```python
from build123d import *

# Parameters (mm, degrees)
SKETCH_1_W          = 5
SKETCH_1_H          = 4
EXTRUDE_1_DEPTH     = 1.5
CHAMFER_1_SIZE      = 0.5
EXTRUDE_2_DEPTH     = 5
SKETCH_3_W          = 0.34
SKETCH_3_H          = 1.1
SKETCH_3_W_2        = 0.76
CUT_EXTRUDE_1_DEPTH = 5.35


with BuildPart() as part:
    # Эскиз1 → Бобышка-Вытянуть1 (new body)
    with BuildSketch(Plane(origin=(0, 0, 0), x_dir=(1, 0, 0), z_dir=(0, 1, 0))):
        Rectangle(SKETCH_1_W, SKETCH_1_H)
    extrude(amount=EXTRUDE_1_DEPTH)

    # Фаска1
    chamfer_1_edges = [part.edges().sort_by_distance(p)[0] for p in [
        (0, 1.5, 2),
    ]]
    chamfer(chamfer_1_edges, length=CHAMFER_1_SIZE)

    # Эскиз2 → Бобышка-Вытянуть2 (add, through all)
    with BuildSketch(Plane(origin=(2.5, 0, 0), x_dir=(0, 0, -1), z_dir=(1, 0, 0))):
        Polygon((-2, 0.75), (-2.25, 0.75), (-2.25, -0.1), (-3.1, -0.1), (-3.1, -0.25), (-2.1, -0.25), (-2.1, 0.6), (0, 0.6), (0, 0.75), align=None)
    extrude_2 = extrude(amount=-EXTRUDE_2_DEPTH)

    # Эскиз3 → Вырез-Вытянуть1 (cut, through all)
    with BuildSketch(Plane(origin=(0, 1.5, 0), x_dir=(1, 0, 0), z_dir=(0, 1, 0))):
        with Locations((-2.33, -2.55)):
            Rectangle(SKETCH_3_W, SKETCH_3_H)
        with Locations((-1.27, -2.55)):
            Rectangle(SKETCH_3_W_2, SKETCH_3_H)
        with Locations((0, -2.55)):
            Rectangle(SKETCH_3_W_2, SKETCH_3_H)
        with Locations((1.27, -2.55)):
            Rectangle(SKETCH_3_W_2, SKETCH_3_H)
        with Locations((2.33, -2.55)):
            Rectangle(SKETCH_3_W, SKETCH_3_H)
    cut_extrude_1 = extrude(amount=-CUT_EXTRUDE_1_DEPTH, mode=Mode.SUBTRACT)

    # Зеркальное отражение1: Бобышка-Вытянуть2, Вырез-Вытянуть1 across plane
    add(extrude_2.mirror(Plane.XY))
    add(cut_extrude_1.mirror(Plane.XY), mode=Mode.SUBTRACT)


solid = part.part
```
For this review, take the finished solid that the model builds, in its own axes (mm). A direction names the side the tool comes from. Round coordinates to 2 decimals unless told otherwise and drop trailing zeros. Write each loop counter-clockwise with the first axis right and the second up, starting at its lowest first coordinate (ties: lowest second). Pieces come first, ordered by that corner, then holes. Notation, with made-up numbers: (79.5, 82) - (127.5, 82) arc R18 ccw to (127.5, 86) - close; hole circle Ø9 at (21, 74). An arc over 180 degrees is marked (long way). Answer as CSV lines item,"result". Start each with the question number.
(1) Add section D-D, the plane y = 1.2. State the section outline as (x, z) points, plus the area to 3 significant figures.
(2) For line 1 (Z direction, x = 2.2, y = 0.6); line 2 (Y direction, x = -0.2, z = 0.5); line 3 (Z direction, x = -1.4, y = 1.45), list the stretches that pass through material, from the lowest coordinate up.
(3) Add section A-A, the plane x = -0.55. State the section outline as (y, z) points, plus the area to 3 significant figures.
(4) For pin 1 (0.8 mm diameter, centred on y = 0, z = -3, fed in from +X); pin 2 (0.5 mm diameter, centred on y = 0, z = -2.5, fed in from -X); pin 3 (0.8 mm diameter, centred on x = -0.5, y = 0.5, fed in from -Z), all flat-tipped, find the tip position at first contact; note any pin that passes through.
(5) Add section C-C, the plane z = -1.5. State the section outline as (x, y) points.
(6) Machinability: for faces 1 (the flat face through (0, 0, 0)), 2 (the flat face through (0, 1.5, 0)), which of the approach directions +Z, -Z, +X, -X, +Y, -Y give a long, thin tool a straight path to every point of the face, cutting with its end or side? Answer none if there is none.
(7) Add section B-B, the plane y = 0.15. State how many separate pieces and enclosed holes the cut face has, plus the area to 3 significant figures.
From the geometry:
1,outline,"(-2.5, -2) - (2.5, -2) - (2.5, 1.8) - (-2.5, 1.8) - close"
1,area,"19.0 mm²"
2,line 1,"z = -2 to 2"
2,line 2,"y = 0 to 1.5"
2,line 3,"z = -2 to 1.55"
3,outline,"(-0.25, -3.1) - (-0.1, -3.1) - (-0.1, -2.25) - (0.75, -2.25) - (0.75, -2) - (1.5, -2) - (1.5, 1.5) - (1, 2) - (0.75, 2) - (0.75, 2.25) - (-0.1, 2.25) - (-0.1, 3.1) - (-0.25, 3.1) - (-0.25, 2.1) - (0.6, 2.1) - (0.6, 2) - (0, 2) - (0, -2) - (0.6, -2) - (0.6, -2.1) - (-0.25, -2.1) - close"
3,area,"6.46 mm²"
4,pin 1,"stops at x = 2.16"
4,pin 2,"stops at x = -2.16"
4,pin 3,"stops at z = -2.25"
5,outline,"(-2.5, 0) - (2.5, 0) - (2.5, 1.5) - (-2.5, 1.5) - close"
6,face 1,"+X, -X, -Y"
6,face 2,"+Z, -Z, +X, -X, +Y"
7,separate pieces,"9"
7,enclosed holes,"0"
7,area,"20.6 mm²"
